from build123d import *

# Parameters (mm, degrees)
BOSS_EXTRUDE1_DEPTH = 8.5
CUT_EXTRUDE1_REACH  = 26.357
SKETCH2_R           = 4
SKETCH3_W           = 2.25
SKETCH3_H           = 10
BOSS_EXTRUDE3_DEPTH = 10
SKETCH4_R           = 5.65
CUT_EXTRUDE2_DEPTH  = 1.5


with BuildPart() as part:
    # Sketch1 → Boss-Extrude1 (new body)
    with BuildSketch(Plane.XY):
        with BuildLine():
            Line((10.712142643, 2.5), (20, 2.5))
            Line((20, 2.5), (20, -2.5))
            Line((20, -2.5), (10.712142643, -2.5))
            ThreePointArc((10.712142643, -2.5), (0, -11), (-10.712142643, -2.5))
            Line((-10.712142643, -2.5), (-20, -2.5))
            Line((-20, -2.5), (-20, 2.5))
            Line((-20, 2.5), (-10.712142643, 2.5))
            ThreePointArc((-10.712142643, 2.5), (0, 11), (10.712142643, 2.5))
        make_face()
    extrude(amount=BOSS_EXTRUDE1_DEPTH)

    # Sketch2 → Cut-Extrude1 (cut, up to next)
    with BuildSketch(Plane.XY.offset(8.5), mode=Mode.PRIVATE) as cut_extrude1_sk1:
        Circle(SKETCH2_R)
    cut_extrude1_tool1 = extrude(cut_extrude1_sk1.sketch, amount=-CUT_EXTRUDE1_REACH, mode=Mode.PRIVATE) & part.part
    add(cut_extrude1_tool1.solids().sort_by_distance((0, 0, 8.5))[0], mode=Mode.SUBTRACT)

    # Sketch3 → Boss-Extrude3 (add)
    with BuildSketch(Plane.XY.offset(8.5)):
        with Locations((7.375, 0)):
            Rectangle(SKETCH3_W, SKETCH3_H)
        with Locations((-7.375, 0)):
            Rectangle(SKETCH3_W, SKETCH3_H)
    extrude(amount=BOSS_EXTRUDE3_DEPTH)

    # Sketch4 → Cut-Extrude2 (cut)
    with BuildSketch(Plane.XY.offset(8.5)):
        Circle(SKETCH4_R)
    extrude(amount=-CUT_EXTRUDE2_DEPTH, mode=Mode.SUBTRACT)


solid = part.part
For this review, take the finished solid that the model builds, in its own axes (mm). A direction names the side the tool comes from. Give positions to 0.01 mm unless a question says otherwise; leave off trailing zeros. Order: outer loops, then holes, each group sorted by start corner. A loop starts at its lowest first (then second) coordinate and runs counter-clockwise, first axis right, second up. Notation, with made-up numbers: (57, 2.25) -> (61, 2.25) arc R7 cw to (61, 13.25) -> close; hole circle Ø1 at (-24, 62). An arc over 180 degrees is marked (long way). Write item = value, one per line.
1) We need section B-B, the plane x = 0. Give the boundary of the cut face in (y, z), and give its area (3 significant figures).
Findings:
outline = (-11, 0) -> (-4, 0) -> (-4, 7) -> (-5.65, 7) -> (-5.65, 8.5) -> (-11, 8.5) -> close; (4, 0) -> (11, 0) -> (11, 8.5) -> (5.65, 8.5) -> (5.65, 7) -> (4, 7) -> close
area = 114 mm^2
2) To check wall thickness, follow L1, parallel to X at y = 2.25, z = 11.5; L2, parallel to Y at x = -7.5, z = 12.5; L3, parallel to Z at x = -6.5, y = -6.25. State the ranges of each line that lie inside material, in increasing order. Write a range as from..to.
Findings:
L1 = -8.5..-6.25, 6.25..8.5
L2 = -5..5
L3 = 0..8.5
3) We need section A-A, the plane z = 14. Give the boundary of the cut face in (x, y).
Findings:
outline = (-8.5, -5) -> (-6.25, -5) -> (-6.25, 5) -> (-8.5, 5) -> close; (6.25, -5) -> (8.5, -5) -> (8.5, 5) -> (6.25, 5) -> close
4) We need section D-D, the plane z = 4.25. Give the boundary of the cut face in (x, y), and give its area (3 significant figures).
Findings:
outline = (-20, -2.5) -> (-10.71, -2.5) arc R11 ccw to (10.71, -2.5) -> (20, -2.5) -> (20, 2.5) -> (10.71, 2.5) arc R11 ccw to (-10.71, 2.5) -> (-20, 2.5) -> close; hole circle Ø8 at (0, 0)
area = 421 mm^2
5) We need section C-C, the plane y = 0. Give the boundary of the cut face in (x, z).
Findings:
outline = (-20, 0) -> (-4, 0) -> (-4, 7) -> (-5.65, 7) -> (-5.65, 8.5) -> (-6.25, 8.5) -> (-6.25, 18.5) -> (-8.5, 18.5) -> (-8.5, 8.5) -> (-20, 8.5) -> close; (4, 0) -> (20, 0) -> (20, 8.5) -> (8.5, 8.5) -> (8.5, 18.5) -> (6.25, 18.5) -> (6.25, 8.5) -> (5.65, 8.5) -> (5.65, 7) -> (4, 7) -> close
6) Draft analysis for pull direction Y (two halves, no side actions). For faces 4 (the face through (-15, 2.5, 4)), 5 (the face through (5.39, 1.7, 7.76)), 6 (the face through (-8.5, 0, 13)), state which applies: pulls with the +Y half, pulls with the -Y half, needs draft (parallel to the pull), parting line crosses it, or undercut.
Findings:
face_4 = pulls with the +Y half
face_5 = undercut
face_6 = needs draft
7) For faces 1 (the face through (7, 5, 13)), 2 (the face through (6.25, 0, 13)), 3 (the face through (-15, -2.5, 4)), list the 3-axis set-ups (+Z, -Z, +X, -X, +Y, -Y) from which the entire face can be reached by the end or side of a thin tool; tool diameter is ignored.
Findings:
face_1 = +Z, +X, -X, +Y
face_2 = +Z, +Y, -Y
face_3 = +Z, -Z, -X, -Y
8) Insertion check: pin 1 (2 mm diameter, centred on x = -9, z = 15.5, fed in from +Y); pin 2 (1 mm diameter, centred on y = 4, z = 14, fed in from +X); pin 3 (3 mm diameter, centred on y = 0.5, z = 15.5, fed in from -X). Each pin has a flat end and moves straight along its axis. Give the tip position at first contact, or say it passes through.
Findings:
pin_1 = 5
pin_2 = 8.5
pin_3 = -8.5
